Geometry: final body of the model. Coordinates: model frame, mm. A direction names the side the tool comes from. Give positions to 0.01 mm unless a question says otherwise; leave off trailing zeros. Order: outer loops, then holes, each group sorted by start corner. A loop starts at its lowest first (then second) coordinate and runs counter-clockwise, first axis right, second up. Notation, with made-up numbers: (31.5, -17) - (84.5, -17) arc R19 ccw to (84.5, -2) - close; hole circle Ø10 at (12, 46). An arc over 180 degrees is marked (long way). Use one line per item in the form item = value.
from build123d import *

# Parameters (mm, degrees)
SKETCH1_W           = 140
SKETCH1_H           = 80
SKETCH1_R           = 2.5
BOSS_EXTRUDE1_DEPTH = 12
FILLET1_R           = 12
SKETCH2_R           = 5.5
CUT_EXTRUDE1_DEPTH  = 6
SKETCH4_R           = 3.25
CUT_EXTRUDE2_DEPTH  = 6
SKETCH5_R           = 2.5
CUT_EXTRUDE3_DEPTH  = 82.510735489


with BuildPart() as part:
    # Sketch1 → Boss-Extrude1 (new body)
    with BuildSketch(Plane(origin=(0, 0, 0), x_dir=(1, 0, 0), z_dir=(0, 1, 0))):
        Rectangle(SKETCH1_W, SKETCH1_H)
        with Locations(Location((22, 21.5, 0), (0, 0, 270))):
            Circle(SKETCH1_R, mode=Mode.SUBTRACT)
        with Locations(Location((47, -3.5, 0), (0, 0, 270))):
            Circle(SKETCH1_R, mode=Mode.SUBTRACT)
        with Locations(Location((-3, -3.5, 0), (0, 0, 270))):
            Circle(SKETCH1_R, mode=Mode.SUBTRACT)
        with Locations(Location((22, -28.5, 0), (0, 0, 270))):
            Circle(SKETCH1_R, mode=Mode.SUBTRACT)
    extrude(amount=BOSS_EXTRUDE1_DEPTH)

    # Fillet1
    fillet1_edges = [part.edges().sort_by_distance(p)[0] for p in [
        (70, 6, 40),
        (-70, 6, 40),
        (-70, 6, -40),
        (70, 6, -40),
    ]]
    fillet(fillet1_edges, radius=FILLET1_R)

    # Sketch2 → Cut-Extrude1 (cut)
    with BuildSketch(Plane(origin=(0, 12, 0), x_dir=(1, 0, 0), z_dir=(0, 1, 0))):
        with Locations(Location((-35, 25, 0), (0, 0, 270))):
            Circle(SKETCH2_R)
        with Locations(Location((-35, -15, 0), (0, 0, 270))):
            Circle(SKETCH2_R)
    extrude(amount=-CUT_EXTRUDE1_DEPTH, mode=Mode.SUBTRACT)

    # Sketch4 → Cut-Extrude2 (cut)
    with BuildSketch(Plane(origin=(0, 6, 0), x_dir=(1, 0, 0), z_dir=(0, 1, 0))):
        with Locations(Location((-35, 25, 0), (0, 0, 270))):
            Circle(SKETCH4_R)
        with Locations(Location((-35, -15, 0), (0, 0, 270))):
            Circle(SKETCH4_R)
    extrude(amount=-CUT_EXTRUDE2_DEPTH, mode=Mode.SUBTRACT)

    # Sketch5 → Cut-Extrude3 (cut, through all)
    with BuildSketch(Plane(origin=(0, 12, 0), x_dir=(1, 0, 0), z_dir=(0, 1, 0))):
        with Locations(Location((-35, 15, 0), (0, 0, 270))):
            Circle(SKETCH5_R)
        with Locations(Location((-35, -5, 0), (0, 0, 270))):
            Circle(SKETCH5_R)
    extrude(amount=-CUT_EXTRUDE3_DEPTH, mode=Mode.SUBTRACT)


solid = part.part
(1) Ray query, line 1 along X through (y, z) = (3.25, -15); line 2 along X through (y, z) = (4, 28.5); line 3 along X through (y, z) = (7, -21.5). Return the intervals inside material, ascending.
Computed values:
line_1 = -70 to -37.5, -32.5 to 70
line_2 = -69.99 to 19.5, 24.5 to 69.99
line_3 = -70 to -39.24, -30.76 to 19.5, 24.5 to 70
(2) Contact query for a flat-ended pin moving along its axis: pin 1 Ø9 at (x, z) = (-35, -25) entering from +Y. Output: stop coordinate, or through.
Computed values:
pin_1 = 6
(3) Cut plane B-B on y = 7.5. Give the number of separate pieces and of enclosed holes in the cut face, plus the area to 3 significant figures.
Computed values:
separate_pieces = 1
enclosed_holes = 8
area = 10,800 mm²
(4) Cut plane C-C on x = 22. Output: boundary loops of the cut face in (y, z), plus the area to 3 significant figures.
Computed values:
outline = (0, -40) - (12, -40) - (12, -24) - (0, -24) - close; (0, -19) - (12, -19) - (12, 26) - (0, 26) - close; (0, 31) - (12, 31) - (12, 40) - (0, 40) - close
area = 840 mm²
(5) Cut plane D-D on x = -35. Output: boundary loops of the cut face in (y, z), plus the area to 3 significant figures.
Computed values:
outline = (0, -40) - (12, -40) - (12, -30.5) - (6, -30.5) - (6, -28.25) - (0, -28.25) - close; (0, -21.75) - (6, -21.75) - (6, -19.5) - (12, -19.5) - (12, -17.5) - (0, -17.5) - close; (0, -12.5) - (12, -12.5) - (12, 2.5) - (0, 2.5) - close; (0, 7.5) - (12, 7.5) - (12, 9.5) - (6, 9.5) - (6, 11.75) - (0, 11.75) - close; (0, 18.25) - (6, 18.25) - (6, 20.5) - (12, 20.5) - (12, 40) - (0, 40) - close
area = 630 mm²
(6) Pull-direction query (Z, two-part tool) for faces 3 (the face through (-30.362, 9.042, -22.043)), 4 (the face through (-32.89, 6.08, 6.34)), 5 (the face through (-1, 6, -40)), 6 (the face through (-1, 6, 40)); classes: released by +Z, released by -Z, zero draft, split by the parting line, or undercut.
Computed values:
face_3 = undercut
face_4 = undercut
face_5 = released by -Z
face_6 = released by +Z
(7) Cut plane A-A on z = 15. Output: boundary loops of the cut face in (x, y), plus the area to 4 significant figures.
Computed values:
outline = (-70, 0) - (-38.25, 0) - (-38.25, 6) - (-40.5, 6) - (-40.5, 12) - (-70, 12) - close; (-31.75, 0) - (70, 0) - (70, 12) - (-29.5, 12) - (-29.5, 6) - (-31.75, 6) - close
area = 1,575 mm²
(8) Reachability of faces 1 (the face through (-39, 6, -25)), 2 (the face through (24, 6, -23)) from +Z, -Z, +X, -X, +Y, -Y: full face, straight path, thin tool, end or side. Return the list, or none.
Computed values:
face_1 = +Y
face_2 = +Y, -Y
